Source: CAD feature listing. Evaluate the final solid. Frame: model axes, mm. Coordinates: 2 decimals unless noted, no trailing zeros. Write each loop counter-clockwise with the first axis right and the second up, starting at its lowest first coordinate (ties: lowest second). Pieces come first, ordered by that corner, then holes. Notation, with made-up numbers: (76, -27) -> (95, -27) arc R14 cw to (95, -12) -> close; hole circle Ø6 at (7.5, 4). An arc over 180 degrees is marked (long way). One line per item, written item: value. Start each with the question number.
1. Section query D-D, the plane x = 42. Output: boundary loops of the cut face in (y, z).
2. Line query: line 1 (X direction, y = 4.66, z = 3.45); line 2 (X direction, y = 6, z = 0.8); line 3 (Y direction, x = 4.18, z = 1.6). Output: solid intervals per line, ascending.
3. Section query A-A, the plane x = 4.18. Output: boundary loops of the cut face in (y, z).
4. Section query B-B, the plane y = 5.5. Output: boundary loops of the cut face in (x, z).
5. Section query C-C, the plane z = 2.6. Output: boundary loops of the cut face in (x, y).
6. Mould query, pull axis Y, two halves, no side actions, for faces 1 (the flat face through (22, 0, 3)), 2 (the flat face through (0, 5, 3)), 3 (the cylindrical face through (32.294, 5.235, 2.953)). Classes: released by +Y, released by -Y, zero draft, split by the parting line, or undercut.
from build123d import *

# Parameters (mm, degrees)
CROQUIS1_W              = 45.16
CROQUIS1_H              = 9.32
CROQUIS1_R              = 1.5
SALIENTE_EXTRUIR1_DEPTH = 5.99


with BuildPart() as part:
    # Croquis1 → Saliente-Extruir1 (new body)
    with BuildSketch(Plane.XY):
        with Locations((22.58, 4.66)):
            Rectangle(CROQUIS1_W, CROQUIS1_H)
        with Locations(Location((4.18, 4.66, 0), (0, 0, 180))):
            Circle(CROQUIS1_R, mode=Mode.SUBTRACT)
        with Locations(Location((11.48, 4.66, 0), (0, 0, 180))):
            Circle(CROQUIS1_R, mode=Mode.SUBTRACT)
        with Locations(Location((40.98, 4.66, 0), (0, 0, 180))):
            Circle(CROQUIS1_R, mode=Mode.SUBTRACT)
        with Locations(Location((33.68, 4.66, 0), (0, 0, 180))):
            Circle(CROQUIS1_R, mode=Mode.SUBTRACT)
    extrude(amount=SALIENTE_EXTRUIR1_DEPTH)


solid = part.part
Computed values:
1. outline: (0, 0) -> (3.56, 0) -> (3.56, 5.99) -> (0, 5.99) -> close; (5.76, 0) -> (9.32, 0) -> (9.32, 5.99) -> (5.76, 5.99) -> close
2. line 1: x = 0 to 2.68, 5.68 to 9.98, 12.98 to 32.18, 35.18 to 39.48, 42.48 to 45.16
2. line 2: x = 0 to 3.51, 4.85 to 10.81, 12.15 to 33.01, 34.35 to 40.31, 41.65 to 45.16
2. line 3: y = 0 to 3.16, 6.16 to 9.32
3. outline: (0, 0) -> (3.16, 0) -> (3.16, 5.99) -> (0, 5.99) -> close; (6.16, 0) -> (9.32, 0) -> (9.32, 5.99) -> (6.16, 5.99) -> close
4. outline: (0, 0) -> (2.94, 0) -> (2.94, 5.99) -> (0, 5.99) -> close; (5.42, 0) -> (10.24, 0) -> (10.24, 5.99) -> (5.42, 5.99) -> close; (12.72, 0) -> (32.44, 0) -> (32.44, 5.99) -> (12.72, 5.99) -> close; (34.92, 0) -> (39.74, 0) -> (39.74, 5.99) -> (34.92, 5.99) -> close; (42.22, 0) -> (45.16, 0) -> (45.16, 5.99) -> (42.22, 5.99) -> close
5. outline: (0, 0) -> (45.16, 0) -> (45.16, 9.32) -> (0, 9.32) -> close; hole circle Ø3 at (4.18, 4.66); hole circle Ø3 at (11.48, 4.66); hole circle Ø3 at (33.68, 4.66); hole circle Ø3 at (40.98, 4.66)
6. face 1: released by -Y
6. face 2: zero draft
6. face 3: undercut
